Verification items for the finished model (mm, model axes). A direction names the side the tool comes from. Give positions to 0.01 mm unless a question says otherwise; leave off trailing zeros. Write each loop counter-clockwise with the first axis right and the second up, starting at its lowest first coordinate (ties: lowest second). Pieces come first, ordered by that corner, then holes. Notation, with made-up numbers: M -36,27 L 16,27 A26 cw 16,48 Z; hole C 33.5,-10.75 d5. An arc over 180 degrees is marked long. Write item = value, one per line.
from build123d import *

# Parameters (mm, degrees)
SKETCH1_W           = 33.54
SKETCH1_H           = 144.78
BOSS_EXTRUDE1_DEPTH = 5.08
SKETCH2_W           = 20.32
SKETCH2_H           = 5.08
BOSS_EXTRUDE2_DEPTH = 5.08
SKETCH3_W           = 20.63
SKETCH3_H           = 5.08
BOSS_EXTRUDE3_DEPTH = 5.08


with BuildPart() as part:
    # Sketch1 → Boss-Extrude1 (new body)
    with BuildSketch(Plane(origin=(0, 0, 0), x_dir=(1, 0, 0), z_dir=(0, 1, 0))):
        with Locations((-16.77, 72.39)):
            Rectangle(SKETCH1_W, SKETCH1_H)
    extrude(amount=BOSS_EXTRUDE1_DEPTH)

    # Sketch2 → Boss-Extrude2 (add)
    with BuildSketch(Plane(origin=(0, 0, -144.78), x_dir=(-1, 0, 0), z_dir=(0, 0, -1))):
        with Locations((16.77, 2.54)):
            Rectangle(SKETCH2_W, SKETCH2_H)
    extrude(amount=BOSS_EXTRUDE2_DEPTH)

    # Sketch3 → Boss-Extrude3 (add)
    with BuildSketch(Plane.XY):
        with Locations((-16.77, 2.54)):
            Rectangle(SKETCH3_W, SKETCH3_H)
    extrude(amount=BOSS_EXTRUDE3_DEPTH)


solid = part.part
1) Draft check along Z on faces 4 (the flat face through (-3, 3, 0)), 5 (the flat face through (-17, 0, -73)), 6 (the flat face through (-3, 3, -144.78)). Enter one of: +Z half, -Z half, draft (parallel to the pull), parting line (faces both ways), or undercut.
From the geometry:
face_4 = +Z half
face_5 = draft
face_6 = -Z half
2) Material ranges on probe 1 along Z at (x, y) = (-28, 3.1); probe 2 along Z at (x, y) = (-6.5, 1.45), recorded low to high. Write a range as from..to.
From the geometry:
probe_1 = -144.78..0
probe_2 = -144.78..5.08
3) Cross-section at A-A on y = 2. Record the boundary of the cut face in (x, z) (3 decimals).
From the geometry:
outline = M -33.54,-144.78 L -26.93,-144.78 L -26.93,-149.86 L -6.61,-149.86 L -6.61,-144.78 L 0,-144.78 L 0,0 L -6.455,0 L -6.455,5.08 L -27.085,5.08 L -27.085,0 L -33.54,0 Z
4) Cross-section at B-B on x = -3. Record the boundary of the cut face in (y, z), plus the area to 3 significant figures.
From the geometry:
outline = M 0,-144.78 L 5.08,-144.78 L 5.08,0 L 0,0 Z
area = 735 mm^2
5) Depth check by flat-ended pin: P1, Ø1.5, axis at x = -29.5, y = 1.5, coming from the -Z side. Enter the tip coordinate at first touch or a pass-through.
From the geometry:
P1 = -144.78
6) Tool access check on faces 1 (the flat face through (-6.61, 3, -147)), 2 (the flat face through (-27.085, 3, 3)), 3 (the flat face through (-26.93, 3, -147)). Record the directions out of +Z, -Z, +X, -X, +Y, -Y that give a thin tool (end or side, any length) a straight path to the whole face; none if there is none.
From the geometry:
face_1 = -Z, +X, +Y, -Y
face_2 = +Z, -X, +Y, -Y
face_3 = -Z, -X, +Y, -Y
